from build123d import *

# Parameters (mm, degrees)
SKETCH1_W               = 11.811
SKETCH1_H               = 45.98924
BOSS_EXTRUDE1_DEPTH     = 9.652
FILLET5_R               = 4.826
SKETCH2_W               = 7.62
SKETCH2_H               = 22.352
CUT_EXTRUDE1_DEPTH      = 7.62
CUT_EXTRUDE2_DEPTH      = 49.452771033
CUT_EXTRUDE2_DEPTH_BACK = 49.452771033
SKETCH3_R               = 2.20345
FILLET4_R               = 4.826
FILLET6_R               = 10.16
CUT_EXTRUDE3_DEPTH      = 49.452771033
CUT_EXTRUDE4_DEPTH      = 7.62
BOSS_EXTRUDE2_DEPTH     = 7.62


with BuildPart() as part:
    # Sketch1 → Boss-Extrude1 (new body)
    with BuildSketch(Plane.XY):
        with Locations((5.9055, 22.99462)):
            Rectangle(SKETCH1_W, SKETCH1_H)
    extrude(amount=BOSS_EXTRUDE1_DEPTH)

    # Fillet5
    fillet5_edges = [part.edges().sort_by_distance(p)[0] for p in [
        (5.9055, 45.98924, 0),
    ]]
    fillet(fillet5_edges, radius=FILLET5_R)

    # Sketch2 → Cut-Extrude1 (cut)
    with BuildSketch(Plane(origin=(0, 0, 0), x_dir=(-1, 0, 0), z_dir=(0, 0, -1))):
        with Locations((-5.9055, 34.81324)):
            Rectangle(SKETCH2_W, SKETCH2_H)
    extrude(amount=-CUT_EXTRUDE1_DEPTH, mode=Mode.SUBTRACT)

    # Sketch3 → Cut-Extrude2 (cut, two sides: drawn at the far end of the back side and taken through both)
    with BuildSketch(Plane.ZY.offset(-CUT_EXTRUDE2_DEPTH_BACK)):
        with Locations((4.4323, 26.82494)):
            Circle(SKETCH3_R)
    extrude(amount=CUT_EXTRUDE2_DEPTH + CUT_EXTRUDE2_DEPTH_BACK, mode=Mode.SUBTRACT)

    # Fillet4
    # the kernel refuses this fillet: 4.826 mm, written as the material it takes off along each edge
    with BuildSketch(Plane(origin=(23.876, 45.98924, 9.652), x_dir=(0, 0, -1), z_dir=(-1, 0, 0))) as fillet4_piece_1:
        with BuildLine():
            CenterArc((FILLET4_R, FILLET4_R), FILLET4_R, 180, 90)
            Line((0, FILLET4_R), (0, 0))
            Line((0, 0), (FILLET4_R, 0))
        make_face()
    extrude(amount=35.941, mode=Mode.SUBTRACT)

    # Fillet6
    # the kernel refuses this fillet: 10.16 mm, written as the material it takes off along each edge
    with BuildSketch(Plane(origin=(-25.368230131, 0, 9.652), x_dir=(0, 1, 0), z_dir=(1, 0, 0))) as fillet6_piece_1:
        with BuildLine():
            CenterArc((10.147292053, -10.16), FILLET6_R, 90, 87.134016017)
            Line((0, -9.652), (-0.202945841, -9.64184))
            ThreePointArc((-0.202945841, -9.64184), (-0.2032, -4.826), (-0.2032, 0))
            Line((-0.2032, 0), (0, 0.2032))
            Line((0, 0.2032), (10.147292053, 0.2032))
            Line((10.147292053, 0.2032), (10.147292053, 0))
        make_face()
    extrude(amount=62.547460263, mode=Mode.SUBTRACT)

    # Sketch4 → Cut-Extrude3 (cut, through all)
    with BuildSketch(Plane(origin=(11.811, 0, 0), x_dir=(0, 0, -1), z_dir=(1, 0, 0))):
        Polygon((-9.652, 35.293813088), (-7.62, 39.52494), (0, 39.52494), (0, 45.98924), (-9.652, 45.98924), align=None)
    extrude(amount=-CUT_EXTRUDE3_DEPTH, mode=Mode.SUBTRACT)

    # Sketch5 → Cut-Extrude4 (cut)
    with BuildSketch(Plane.ZY.offset(-9.7155)):
        Polygon((0, 21.160076085), (5.158068358, 23.63724), (0, 23.63724), align=None)
    extrude(amount=CUT_EXTRUDE4_DEPTH, mode=Mode.SUBTRACT)

    # Sketch5<3> → Boss-Extrude2 (add)
    with BuildSketch(Plane.ZY.offset(-9.7155)):
        with BuildLine():
            Line((5.812301369, 23.951435604), (5.158068358, 23.63724))
            Line((5.158068358, 23.63724), (7.62, 23.63724))
            Line((7.62, 23.63724), (7.62, 26.82494))
            ThreePointArc((7.62, 26.82494), (7.130490287, 25.127530072), (5.812301369, 23.951435604))
        make_face()
    extrude(amount=BOSS_EXTRUDE2_DEPTH)


solid = part.part
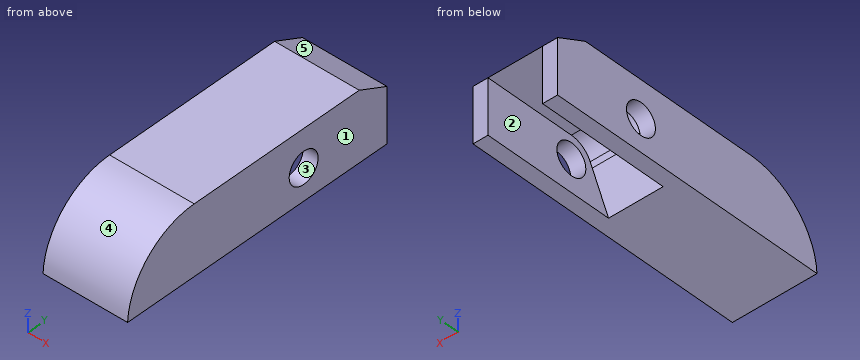
Verification items for the finished model (mm, model axes). Face numbers are marked on the shaded views. A direction names the side the tool comes from. Give positions to 0.01 mm unless a question says otherwise; leave off trailing zeros. Order: outer loops, then holes, each group sorted by start corner. A loop starts at its lowest first (then second) coordinate and runs counter-clockwise, first axis right, second up. Notation, with made-up numbers: M 63,-1 L 105,-1 A30 ccw 105,29 Z; hole C -2.75,2.25 d7. An arc over 180 degrees is marked long. Answer as a JSON object with one key per item and string values. Group by question number.
1) Depth check by flat-ended pin: pin 1 Ø1 at (x, z) = (3, 5.5) entering from +Y; pin 2 Ø1 at (x, z) = (10, 2) entering from -Y; pin 3 Ø5 at (y, z) = (7, 6) entering from -X; pin 4 Ø4 at (x, y) = (5.5, 36) entering from -Z. Enter the tip coordinate at first touch or a pass-through.
2) Cross-section at D-D (x = 3). Enter the section's corners in (y, z), then the cut area to 3 significant figures.
3) Cross-section at B-B (y = 34). Enter the section's corners in (x, z), then the cut area to 3 significant figures.
4) Cross-section at A-A (z = 4.25). Enter the section's corners in (x, y), then the cut area to 3 significant figures.
5) Mould release check, pull along Y, two halves, no side actions. Record for the marked faces 3, 4 and 5: released by +Y, released by -Y, zero draft, split by the parting line, or undercut.
6) Access from +Z, -Z, +X, -X, +Y, -Y to the whole of each face (thin tool, end or side, straight path). Record for the marked faces 1 and 2.
7) Cross-section at C-C (x = 10.25). Enter the section's corners in (y, z).
8) Scan lines: line 1 along X through (y, z) = (24.5, 5.75); line 2 along Y through (x, z) = (10.5, 5.5); line 3 along Z through (x, y) = (4, 31.5). Record each from-to range of solid material in increasing order. Write a range as [from, to].
Result sheet:
{
 "1": {"pin 1": "stops at y = 24.05", "pin 2": "stops at y = 0.19", "pin 3": "stops at x = 0", "pin 4": "stops at z = 7.62"},
 "2": {"outline": "M 0,0 L 21.16,0 L 23.95,5.81 A3.19 cw 26.82,7.62 L 39.52,7.62 L 35.29,9.65 L 10.15,9.65 A10.16 ccw Z", "area": "230 mm2"},
 "3": {"outline": "M 0,0 L 2.1,0 L 2.1,7.62 L 9.72,7.62 L 9.72,0 L 11.81,0 L 11.81,9.65 L 0,9.65 Z", "area": "55.9 mm2"},
 "4": {"outline": "M 0,1.17 L 11.81,1.17 L 11.81,24.63 L 9.72,24.63 L 9.72,23.2 L 2.1,23.2 L 2.1,24.63 L 0,24.63 Z; M 0,29.02 L 2.1,29.02 L 2.1,39.52 L 0,39.52 Z; M 9.72,29.02 L 11.81,29.02 L 11.81,39.52 L 9.72,39.52 Z", "area": "310 mm2"},
 "5": {"face 3": "undercut", "face 4": "released by -Y", "face 5": "released by +Y"},
 "6": {"face 1": "+Z, -Z, +X, +Y, -Y", "face 2": "-Z, +Y"},
 "7": {"outline": "M 0,0 L 39.52,0 L 39.52,7.62 L 35.29,9.65 L 10.15,9.65 A10.16 ccw Z; hole C 26.82,4.43 d4.41"},
 "8": {"line 1": "x = [0, 2.1], [9.72, 11.81]", "line 2": "y = [1.95, 24.9], [28.75, 39.52]", "line 3": "z = [7.62, 9.65]"}
}
